Source: three-view drawing plus pictorial views. Frame: mm from the lowest corner of the part. A direction names the side the tool comes from. Round coordinates to 2 decimals unless told otherwise and drop trailing zeros. Loops run counter-clockwise (first coordinate to the right, second up) from the corner with the lowest first, then second, coordinate; pieces in that order, holes last. Notation, with made-up numbers: (71.25, 62) -> (115.25, 62) arc R30 cw to (115.25, 94) -> close; hole circle Ø7 at (-25.5, 65). An arc over 180 degrees is marked (long way). Answer as a JSON object with one key per item and string values. Group by question number.
Item 1: Set-up query: the marked faces 4 and 5. Return all of +Z, -Z, +X, -X, +Y, -Y with unobstructed straight access to the full face (end or side cutting, diameter ignored); none if empty.
Item 2: Pin query (flat end, axial travel): pin 1 (3 mm diameter, centred on x = 26.5, z = 4, fed in from +Y); pin 2 (1.5 mm diameter, centred on x = 28, z = 1.5, fed in from +Y); pin 3 (3 mm diameter, centred on y = 27.5, z = 5.5, fed in from -X) (1 decimal). Return the tip coordinate at first contact, or that it passes through.
Item 3: Draft query along X for the marked faces 1, 2 and 3. Return one class per face: released by +X, released by -X, zero draft, split by the parting line, or undercut.
Item 4: Section query D-D on x = 4.5. Return loops of the section in (y, z).
Item 5: Section query B-B on x = 18. Return loops of the section in (y, z).
Item 6: Material intervals for line 1 (Y direction, x = 17.5, z = 1); line 2 (X direction, y = 21, z = 8.25); line 3 (X direction, y = 23, z = 9.5), sorted ascending. Write a range as [from, to].
Item 7: Section query A-A on z = 7.25. Return loops of the section in (x, y).
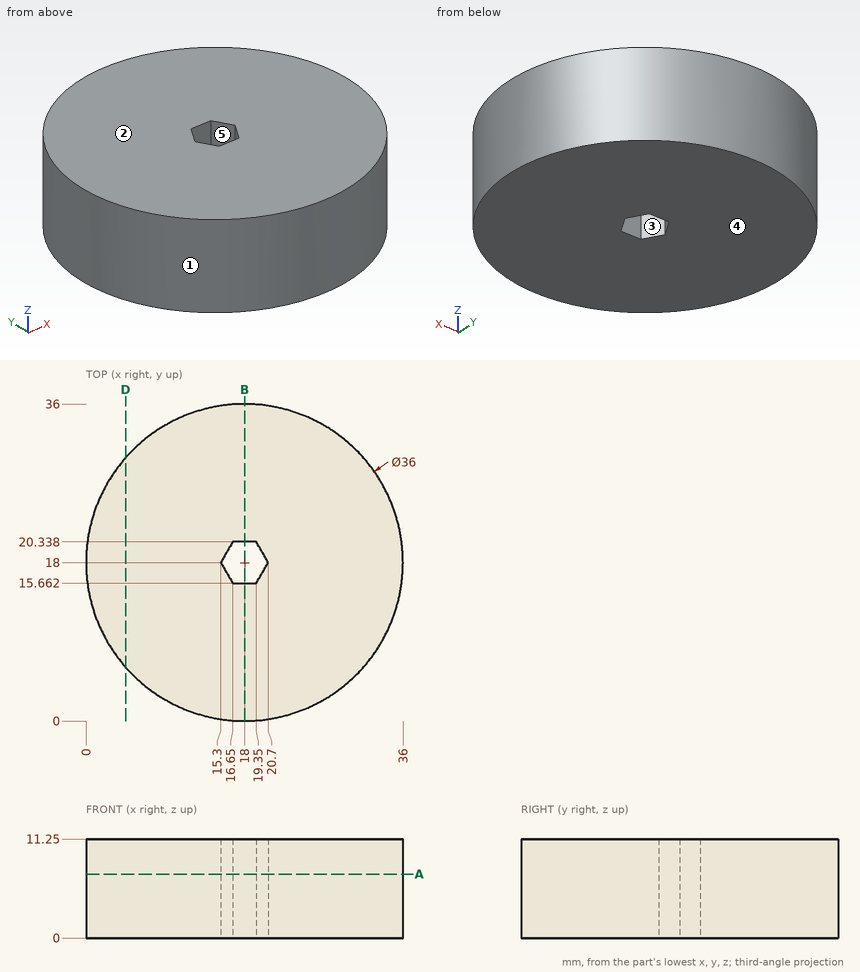
Solved:
{
 "1": {"face 4": "-Z, +X, -X, +Y, -Y", "face 5": "+Z, -Z"},
 "2": {"pin 1": "y = 34.58", "pin 2": "y = 33.44", "pin 3": "x = 1.9"},
 "3": {"face 1": "split by the parting line", "face 2": "zero draft", "face 3": "undercut"},
 "4": {"outline": "(6.09, 0) -> (29.91, 0) -> (29.91, 11.25) -> (6.09, 11.25) -> close"},
 "5": {"outline": "(0, 0) -> (15.66, 0) -> (15.66, 11.25) -> (0, 11.25) -> close; (20.34, 0) -> (36, 0) -> (36, 11.25) -> (20.34, 11.25) -> close"},
 "6": {"line 1": "[0.01, 15.66], [20.34, 35.99]", "line 2": "[0.25, 35.75]", "line 3": "[0.71, 35.29]"},
 "7": {"outline": "circle Ø36 at (18, 18); hole (15.3, 18) -> (16.65, 15.66) -> (19.35, 15.66) -> (20.7, 18) -> (19.35, 20.34) -> (16.65, 20.34) -> close"}
}
